from build123d import *

# Parameters (mm, degrees)
SKETCH1_W           = 91.44
SKETCH1_H           = 6.35
BOSS_EXTRUDE1_DEPTH = 32.131
SKETCH2_R           = 1.1303
CUT_EXTRUDE1_DEPTH  = 12.7


with BuildPart() as part:
    # Sketch1 → Boss-Extrude1 (new body)
    with BuildSketch(Plane(origin=(0, 0, 0), x_dir=(1, 0, 0), z_dir=(0, 1, 0))):
        with Locations((-45.72, -3.175)):
            Rectangle(SKETCH1_W, SKETCH1_H)
    extrude(amount=BOSS_EXTRUDE1_DEPTH)

    # Sketch2 → Cut-Extrude1 (cut)
    with BuildSketch(Plane(origin=(0, 0, 0), x_dir=(0, 0, -1), z_dir=(1, 0, 0))):
        with Locations((-3.175, 28.956)):
            Circle(SKETCH2_R)
    cut_extrude1 = extrude(amount=-CUT_EXTRUDE1_DEPTH, mode=Mode.SUBTRACT)

    # Mirror1: Cut-Extrude1 across plane
    add(cut_extrude1.mirror(Plane(origin=(-45.72, 0, 0), x_dir=(0, 0, 1), z_dir=(1, 0, 0))), mode=Mode.SUBTRACT)


solid = part.part
For this review, take the finished solid that the model builds, in its own axes (mm). A direction names the side the tool comes from. Coordinates: 2 decimals unless noted, no trailing zeros. Order: outer loops, then holes, each group sorted by start corner. A loop starts at its lowest first (then second) coordinate and runs counter-clockwise, first axis right, second up. Notation, with made-up numbers: (37, 40.5) - (78, 40.5) arc R14 ccw to (78, 63.5) - close; hole circle Ø6 at (17.5, 7). An arc over 180 degrees is marked (long way). Use one line per item in the form item = value.
Q1. Draft analysis for pull direction Y (two halves, no side actions). For faces 1 (the cylindrical face through (-85.179, 27.953, 2.653)), 2 (the flat face through (-46, 0, 3)), 3 (the flat face through (-46, 16, 6.35)), state which applies: +Y half, -Y half, draft (parallel to the pull), parting line (faces both ways), or undercut.
Checked values:
face_1 = undercut
face_2 = -Y half
face_3 = draft
Q2. For faces 4 (the flat face through (0, 16, 3)), 5 (the flat face through (-12.7, 29, 3)), 6 (the flat face through (-78.74, 29, 3)), list the 3-axis set-ups (+Z, -Z, +X, -X, +Y, -Y) from which the entire face can be reached by the end or side of a thin tool; tool diameter is ignored.
Checked values:
face_4 = +Z, -Z, +X, +Y, -Y
face_5 = +X
face_6 = -X
Q3. Consider section B-B (x = -10). Give the boundary of the cut face in (y, z) (3 decimals), then the cut area to 3 significant figures.
Checked values:
outline = (0, 0) - (32.131, 0) - (32.131, 6.35) - (0, 6.35) - close; hole circle Ø2.261 at (28.956, 3.175)
area = 200 mm2
Q4. For P1, Ø1.8, axis at y = 28.956, z = 3.175, coming from the -X side, flat-tipped, find the tip position at first contact; note if it passes through.
Checked values:
P1 = -78.74
Q5. Consider section A-A (z = 3.25). Give the boundary of the cut face in (x, y), then the cut area to 3 significant figures.
Checked values:
outline = (-91.44, 0) - (0, 0) - (0, 27.83) - (-12.7, 27.83) - (-12.7, 30.08) - (0, 30.08) - (0, 32.13) - (-91.44, 32.13) - (-91.44, 30.08) - (-78.74, 30.08) - (-78.74, 27.83) - (-91.44, 27.83) - close
area = 2,880 mm2
